```python
from build123d import *

# Parameters (mm, degrees)
F2_DEPTH = 25
F3_DEPTH = 20
F4_DEPTH = 25


with BuildPart() as f2:
    # F1 (on Top) → F2 (new body)
    with BuildSketch(Plane.XY):
        with BuildLine():
            ThreePointArc((-8.8167787844, 7.1352549156), (-13.4599944512, 5.0779075669), (-18.5244405716, 4.6990733883))
            Line((-18.5244405716, 4.6990733883), (-19.36615562, 4.9725631861))
            ThreePointArc((-19.36615562, 4.9725631861), (-23.7764129074, 2.7254248594), (-21.5292745807, -1.684832428))
            Line((-21.5292745807, -1.684832428), (-20.6875595323, -1.9583222258))
            ThreePointArc((-20.6875595323, -1.9583222258), (-16.813009697, -5.241612255), (-14.2658477444, -9.6352549156))
            ThreePointArc((-14.2658477444, -9.6352549156), (-13.7440266917, -14.6869707262), (-14.9487338959, -19.6206114097))
            Line((-14.9487338959, -19.6206114097), (-15.4689424046, -20.336616996))
            ThreePointArc((-15.4689424046, -20.336616996), (-14.6946313073, -25.2254248594), (-9.805823444, -24.4511137621))
            Line((-9.805823444, -24.4511137621), (-9.2856149352, -23.7351081758))
            ThreePointArc((-9.2856149352, -23.7351081758), (-4.9657188134, -21.0647847237), (0, -20))
            ThreePointArc((0, -20), (4.9657188134, -21.0647847237), (9.2856149352, -23.7351081758))
            Line((9.2856149352, -23.7351081758), (9.805823444, -24.4511137621))
            ThreePointArc((9.805823444, -24.4511137621), (14.6946313073, -25.2254248594), (15.4689424046, -20.336616996))
            Line((15.4689424046, -20.336616996), (14.9487338959, -19.6206114097))
            ThreePointArc((14.9487338959, -19.6206114097), (13.7440266917, -14.6869707262), (14.2658477444, -9.6352549156))
            ThreePointArc((14.2658477444, -9.6352549156), (16.813009697, -5.241612255), (20.6875595323, -1.9583222258))
            Line((20.6875595323, -1.9583222258), (21.5292745807, -1.684832428))
            ThreePointArc((21.5292745807, -1.684832428), (23.7764129074, 2.7254248594), (19.36615562, 4.9725631861))
            Line((19.36615562, 4.9725631861), (18.5244405716, 4.6990733883))
            ThreePointArc((18.5244405716, 4.6990733883), (13.4599944512, 5.0779075669), (8.8167787844, 7.1352549156))
            ThreePointArc((8.8167787844, 7.1352549156), (5.4252926325, 10.915460138), (3.5, 15.614968423))
            Line((3.5, 15.614968423), (3.5, 16.5))
            ThreePointArc((3.5, 16.5), (0, 20), (-3.5, 16.5))
            Line((-3.5, 16.5), (-3.5, 15.614968423))
            ThreePointArc((-3.5, 15.614968423), (-5.4252926325, 10.915460138), (-8.8167787844, 7.1352549156))
        make_face()
    extrude(amount=F2_DEPTH)

    # F0 (on Top) → F3 (join)
    with BuildSketch(Plane.XY):
        with BuildLine():
            ThreePointArc((16.164094438, -27.2479673453), (24.5026794152, -17.4847387428), (27.5, -5))
            ThreePointArc((27.5, -5), (27.1614293664, -0.6980522114), (26.1540541981, 3.4979673453))
            Line((26.1540541981, 3.4979673453), (23.7764129074, 2.7254248594))
            Line((23.7764129074, 2.7254248594), (0, -5))
            Line((0, -5), (14.6946313073, -25.2254248594))
            Line((14.6946313073, -25.2254248594), (16.164094438, -27.2479673453))
        make_face()
        with BuildLine():
            Line((23.7764129074, 2.7254248594), (26.1540541981, 3.4979673453))
            ThreePointArc((26.1540541981, 3.4979673453), (0, 22.5), (-26.1540541981, 3.4979673453))
            Line((-26.1540541981, 3.4979673453), (-23.7764129074, 2.7254248594))
            Line((-23.7764129074, 2.7254248594), (0, -5))
            Line((0, -5), (23.7764129074, 2.7254248594))
        make_face()
        with BuildLine():
            ThreePointArc((-16.164094438, -27.2479673453), (0, -32.5), (16.164094438, -27.2479673453))
            Line((16.164094438, -27.2479673453), (14.6946313073, -25.2254248594))
            Line((14.6946313073, -25.2254248594), (0, -5))
            Line((0, -5), (-14.6946313073, -25.2254248594))
            Line((-14.6946313073, -25.2254248594), (-16.164094438, -27.2479673453))
        make_face()
        with BuildLine():
            Line((-23.7764129074, 2.7254248594), (-26.1540541981, 3.4979673453))
            ThreePointArc((-26.1540541981, 3.4979673453), (-26.1540541981, -13.4979673453), (-16.164094438, -27.2479673453))
            Line((-16.164094438, -27.2479673453), (-14.6946313073, -25.2254248594))
            Line((-14.6946313073, -25.2254248594), (0, -5))
            Line((0, -5), (-23.7764129074, 2.7254248594))
        make_face()
    extrude(amount=F3_DEPTH)

    # F4 (cut): a face of the model
    f4_faces = [f2.faces().sort_by_distance(p)[0] for p in [
        (0, -5, 25),
    ]]
    extrude(f4_faces, amount=-F4_DEPTH, mode=Mode.SUBTRACT)


solid = f2.part
```
Geometry: final body of the model. Coordinates: model frame, mm. A direction names the side the tool comes from. Round coordinates to 2 decimals unless told otherwise and drop trailing zeros. Order: outer loops, then holes, each group sorted by start corner. A loop starts at its lowest first (then second) coordinate and runs counter-clockwise, first axis right, second up. Notation, with made-up numbers: (41, -23.75) -> (62, -23.75) arc R18 ccw to (62, 6.25) -> close; hole circle Ø10 at (86.5, 9). An arc over 180 degrees is marked (long way). Write each question's results on one line, items separated by ' | '.
Q1. Section query B-B (z = 10). Output: boundary loops of the cut face in (x, y), and give its area (3 significant figures).
Response values:
outline: circle Ø55 at (0, -5); hole (-21.53, -1.68) -> (-20.69, -1.96) arc R14.9 cw to (-14.27, -9.64) arc R14.9 cw to (-14.95, -19.62) -> (-15.47, -20.34) arc R3.5 ccw to (-9.81, -24.45) -> (-9.29, -23.74) arc R14.9 cw to (0, -20) arc R14.9 cw to (9.29, -23.74) -> (9.81, -24.45) arc R3.5 ccw to (15.47, -20.34) -> (14.95, -19.62) arc R14.9 cw to (14.27, -9.64) arc R14.9 cw to (20.69, -1.96) -> (21.53, -1.68) arc R3.5 ccw to (19.37, 4.97) -> (18.52, 4.7) arc R14.9 cw to (8.82, 7.14) arc R14.9 cw to (3.5, 15.61) -> (3.5, 16.5) arc R3.5 ccw to (-3.5, 16.5) -> (-3.5, 15.61) arc R14.9 cw to (-8.82, 7.14) arc R14.9 cw to (-18.52, 4.7) -> (-19.37, 4.97) arc R3.5 ccw to start | area: 1,250 mm²
Q2. Section query C-C (x = 6). Output: boundary loops of the cut face in (y, z), and give its area (3 significant figures).
Response values:
outline: (-31.84, 0) -> (-21.53, 0) -> (-21.53, 20) -> (-31.84, 20) -> close; (10.07, 0) -> (21.84, 0) -> (21.84, 20) -> (10.07, 20) -> close | area: 442 mm²
Q3. Section query A-A (y = -3.5). Output: boundary loops of the cut face in (x, z).
Response values:
outline: (-27.46, 0) -> (-18.53, 0) -> (-18.53, 20) -> (-27.46, 20) -> close; (18.53, 0) -> (27.46, 0) -> (27.46, 20) -> (18.53, 20) -> close
Q4. Ray query, line 1 along Y through (x, z) = (-15, 15.5); line 2 along Y through (x, z) = (17, 4.25); line 3 along Y through (x, z) = (1, 6). Return the intervals inside material, ascending.
Response values:
line 1: -28.05 to -24.98, -19.69 to -7.97, 4.78 to 18.05 | line 2: -26.62 to -5.02, 4.63 to 16.62 | line 3: -32.48 to -20.07, 19.85 to 22.48
Q5. Pull-direction query (Y, two-part tool) for faces 3 (the face through (18, -5, 20)), 4 (the face through (-23.75, 2.8, 10.14)); classes: released by +Y, released by -Y, zero draft, split by the parting line, or undercut.
Response values:
face 3: zero draft | face 4: undercut
Q6. Access query for faces 1 (the face through (18, -5, 0)), 2 (the face through (13.53, 5.06, 10.14)). Directions: +Z, -Z, +X, -X, +Y, -Y. A direction counts if a zero-diameter tool reaches every point of the face in a straight line with its end or side. Return the directions, or none.
Response values:
face 1: -Z, +X, -X, +Y, -Y | face 2: +Z, -Z
Q7. Pin query (flat end, axial travel): pin 1 Ø3 at (x, z) = (16.5, 13) entering from +Y; pin 2 Ø1.5 at (y, z) = (-24.5, 9.5) entering from -X; pin 3 Ø1 at (y, z) = (16, 6.5) entering from +X. Return the tip coordinate at first contact, or that it passes through.
Response values:
pin 1: y = 18.05 | pin 2: x = -20.12 | pin 3: x = 18.33
